from build123d import *

# Parameters (mm, degrees)
SKETCH1_W           = 63.5
SKETCH1_H           = 6.35
SKETCH1_R           = 1.905
BOSS_EXTRUDE1_DEPTH = 2.54
SKETCH2_W           = 2.54
SKETCH2_H           = 6.35
BOSS_EXTRUDE2_DEPTH = 5.08
SKETCH3_W           = 63.5
SKETCH3_H           = 3.175
CUT_EXTRUDE1_DEPTH  = 3.81


with BuildPart() as part:
    # Sketch1 → Boss-Extrude1 (new body)
    with BuildSketch(Plane(origin=(0, 0, 0), x_dir=(1, 0, 0), z_dir=(0, 1, 0))):
        Rectangle(SKETCH1_W, SKETCH1_H)
        Circle(SKETCH1_R, mode=Mode.SUBTRACT)
        with Locations((-19.05, 0)):
            Circle(SKETCH1_R, mode=Mode.SUBTRACT)
        with Locations((19.05, 0)):
            Circle(SKETCH1_R, mode=Mode.SUBTRACT)
    extrude(amount=BOSS_EXTRUDE1_DEPTH)

    # Sketch2 → Boss-Extrude2 (add)
    with BuildSketch(Plane.XZ):
        with Locations((-9.525, 0)):
            Rectangle(SKETCH2_W, SKETCH2_H)
        with Locations((-28.575, 0)):
            Rectangle(SKETCH2_W, SKETCH2_H)
        with Locations((9.525, 0)):
            Rectangle(SKETCH2_W, SKETCH2_H)
        with Locations((28.575, 0)):
            Rectangle(SKETCH2_W, SKETCH2_H)
    extrude(amount=BOSS_EXTRUDE2_DEPTH)

    # Sketch3 → Cut-Extrude1 (cut)
    with BuildSketch(Plane.XY.offset(3.175)):
        with Locations((0, -1.5875)):
            Rectangle(SKETCH3_W, SKETCH3_H)
    extrude(amount=-CUT_EXTRUDE1_DEPTH, mode=Mode.SUBTRACT)


solid = part.part
Work out the finished part from the listing and answer in its coordinate system (mm). A direction names the side the tool comes from. Round coordinates to 2 decimals unless told otherwise and drop trailing zeros. Write each loop counter-clockwise with the first axis right and the second up, starting at its lowest first coordinate (ties: lowest second). Pieces come first, ordered by that corner, then holes. Notation, with made-up numbers: (70.5, 71) -> (116.5, 71) arc R26 cw to (116.5, 101) -> close; hole circle Ø8 at (-21.75, 55). An arc over 180 degrees is marked (long way). Answer as CSV lines item,"result". Start each with the question number.
(1) Find the intervals of material crossed by probe 1 along X at (y, z) = (-4.25, 1.25) (3 decimals); probe 2 along X at (y, z) = (2.05, 0) (3 decimals); probe 3 along Z at (x, y) = (0, 0.55) (3 decimals), in increasing order.
(2) The part is cut by section B-B, the plane y = -0.75. Give the vertices of the cut face in (x, z) (3 decimals), then the cut area to 3 significant figures.
(3) A tool of negligible diameter and unlimited length cuts with its end or side. For faces 5 (the flat face through (-8.255, -3, -1)), 6 (the flat face through (-0.4, 0, 2.1)), 7 (the flat face through (-10, -2, -0.635)), 8 (the flat face through (29, -5.08, 0)), from which of +Z, -Z, +X, -X, +Y, -Y can it reach the whole face along a straight path? Write none if from no direction.
(4) Each of these flat-tipped pins is pushed along its axis until it touches: pin 1 (1.5 mm diameter, centred on y = -2.5, z = -1.5, fed in from -X) (3 decimals); pin 2 (0.8 mm diameter, centred on x = -28.5, y = -1.5, fed in from +Z) (3 decimals); pin 3 (3 mm diameter, centred on x = -2.5, z = -1.5, fed in from -Y); pin 4 (2.5 mm diameter, centred on x = 0, z = 0, fed in from +Y). Where does it stop, or does it pass through?
(5) The part is cut by section C-C, the plane x = -19.05. Give the vertices of the cut face in (y, z) (3 decimals), then the cut area to 3 significant figures.
(6) The mould has two halves that part along X. Classify faces 1 (the cylindrical face through (17.147, 1.252, -0.084)), 2 (the flat face through (29, -2, -0.635)), 3 (the flat face through (31.75, 1, 0)), 4 (the flat face through (-10.795, -3, -1)): +X half, -X half, draft (parallel to the pull), parting line (faces both ways), or undercut.
(7) The part is cut by section A-A, the plane z = 0. Give the number of separate pieces and of enclosed holes in the cut face, then the cut area to 3 significant figures.
Output values:
1,probe 1,"x = -29.845 to -27.305, -10.795 to -8.255, 8.255 to 10.795, 27.305 to 29.845"
1,probe 2,"x = -31.75 to -20.955, -17.145 to -1.905, 1.905 to 17.145, 20.955 to 31.75"
1,probe 3,"z = -3.175 to -1.905, 1.905 to 3.175"
2,outline,"(-29.845, -3.175) -> (-27.305, -3.175) -> (-27.305, -0.635) -> (-29.845, -0.635) -> close; (-10.795, -3.175) -> (-8.255, -3.175) -> (-8.255, -0.635) -> (-10.795, -0.635) -> close; (8.255, -3.175) -> (10.795, -3.175) -> (10.795, -0.635) -> (8.255, -0.635) -> close; (27.305, -3.175) -> (29.845, -3.175) -> (29.845, -0.635) -> (27.305, -0.635) -> close"
2,area,"25.8 mm²"
3,face 5,"+Z, -Z, -Y"
3,face 6,"+Z"
3,face 7,"+Z, +X, -X"
3,face 8,"+Z, -Z, +X, -X, -Y"
4,pin 1,"stops at x = -29.845"
4,pin 2,"stops at z = -0.635"
4,pin 3,"stops at y = 0"
4,pin 4,"passes through"
5,outline,"(0, -3.175) -> (2.54, -3.175) -> (2.54, -1.905) -> (0, -1.905) -> close; (0, 1.905) -> (2.54, 1.905) -> (2.54, 3.175) -> (0, 3.175) -> close"
5,area,"6.45 mm²"
6,face 1,"undercut"
6,face 2,"draft"
6,face 3,"+X half"
6,face 4,"undercut"
7,separate pieces,"8"
7,enclosed holes,"0"
7,area,"152 mm²"
